For this review, take the finished solid that the model builds, in its own axes (mm). Face numbers are marked on the shaded views. Give positions to 0.01 mm unless a question says otherwise; leave off trailing zeros. Order: outer loops, then holes, each group sorted by start corner. A loop starts at its lowest first (then second) coordinate and runs counter-clockwise, first axis right, second up.
Item 1: Consider section A-A (z = 80.5). Give the boundary of the cut face in (x, y), plus the area to 3 significant figures.
Item 2: Consider section D-D (y = -23). Give the boundary of the cut face in (x, z), plus the area to 3 significant figures.
Item 3: The part is to be moulded in two halves that separate along X. For the marked faces 1, 2 and 3, say which applies: released by +X, released by -X, zero draft, split by the parting line, or undercut.
Item 4: For probe 1 along Y at (x, z) = (-0.25, 115); probe 2 along Z at (x, y) = (-0.75, -17); probe 3 along Z at (x, y) = (-11.25, -7), list the stretches that pass through material, from the lowest coordinate up.
Item 5: For P1, Ø6, axis at x = -1.5, z = 27, coming from the -Y side; P2, Ø5, axis at y = -2, z = 47.5, coming from the +X side; P3, Ø9.5, axis at x = 0, y = 0, coming from the -Z side; P4, Ø8, axis at x = 0.5, y = -3.5, coming from the +Z side, all flat-tipped, find the tip position at first contact; note any pin that passes through.
Item 6: Consider section B-B (x = 0). Give the boundary of the cut face in (y, z).
Item 7: Consider section C-C (y = 0). Give the boundary of the cut face in (x, z).
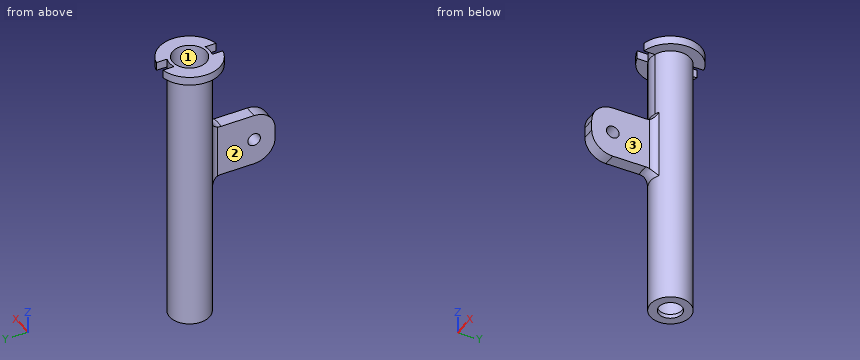
Autodesk Inventor part; units mm, degrees
ref_plane "YZ Plane" through (0, 0, 0) normal (1, 0, 0) x (0, 1, 0)
ref_plane "XZ Plane" through (0, 0, 0) normal (0, 1, 0) x (-1, 0, 0)
ref_plane "XY Plane" through (0, 0, 0) normal (0, 0, 1) x (1, 0, 0)
sketch "Boceto2" plane through (0, 0, 0) normal (0, 0, 1) x (1, 0, 0)
  circle A0 centre (0, 0) radius 9.5
  circle A1 centre (0, 0) radius 5.5
extrude "Extrusión1" add sketch "Boceto2" along normal blind 2
sketch "Boceto3" plane through (0, 0, 2) normal (0, 0, 1) x (1, 0, 0)
  circle A0 centre (0, 0) radius 9.5
  circle A1 centre (0, 0) radius 8
  dimension "d5" = 16
extrude "Extrusión2" add sketch "Boceto3" along normal blind 130
sketch "Boceto4" plane through (0, 0, 132) normal (0, 0, 1) x (1, 0, 0)
  circle A0 centre (0, 0) radius 9.5
  circle A1 centre (0, 0) radius 8
  circle A2 centre (0, 0) radius 14.5
  line L0 (3, 14.186261) -> (3, -14.186261)
  line L1 (-3, 14.186261) -> (-3, -14.186261)
  point P0 (3, 0)
  point P1 (-3, 0)
  point P2 (-3, 9.013878)
  point P3 (-3, -9.013878)
  point P4 (3, -9.013878)
  point P5 (3, 9.013878)
  dimension "d36" = 19
  dimension "d37" = 5
  dimension "d38" = 3
  dimension "d39" = 3
extrude "Extrusión3" add sketch "Boceto4" against normal blind 4 contours A0 L0 A2 | A0 L1 A2
sketch "Boceto5" plane through (0, 0, 128) normal (0, 0, -1) x (-1, 0, 0)
  line L0 (9.380832, 1.5) -> (10.897247, 1.5)
  line L1 (-9.380832, 1.5) -> (-10.897247, 1.5)
  line L2 (-9.380832, -1.5) -> (-10.897247, -1.5)
  line L3 (9.380832, -1.5) -> (10.897247, -1.5)
  arc A0 (-9.380832, 1.5) -> (-9.380832, -1.5) centre (0, 0) ccw
  arc A1 (9.380832, -1.5) -> (9.380832, 1.5) centre (0, 0) ccw
  line L4 (-10.897247, 1.5) -> (-12.409674, 1.5)
  line L5 (-10.897247, -1.5) -> (-12.409674, -1.5)
  line L6 (10.897247, 1.5) -> (12.409674, 1.5)
  line L7 (10.897247, -1.5) -> (12.409674, -1.5)
  arc A2 (-12.409674, 1.5) -> (-12.409674, -1.5) centre (0, 0) ccw
  arc A3 (12.409674, -1.5) -> (12.409674, 1.5) centre (0, 0) ccw
extrude "Extrusión4" [suppressed]
sketch "Boceto6" plane through (0, 0, 128) normal (0, 0, -1) x (-1, 0, 0)
  arc A0 (-3, -9.013878) -> (3, -9.013878) centre (0, 0) ccw
  line L0 (-2.5, -20.682789) -> (-2.5, -15.634719)
  line L1 (-3, -9.013878) -> (-3, -39.013878)
  line L2 (3, -9.013878) -> (3, -39.013878)
  line L3 (-3, -39.013878) -> (3, -39.013878)
  point P0 (-1.5, -10.897247)
  point P1 (-1.5, -9.380832)
extrude "Extrusión5" add sketch "Boceto6" along normal blind 60
sketch "Boceto7" plane through (0, 0, 128) normal (0, 0, 1) x (1, 0, 0)
  line L0 (-3, -39.013878) -> (-3, -9.013878)
  line L1 (-3, -9.013878) -> (-3, -39.013878)
  line L2 (3, -39.013878) -> (-3, -39.013878)
  line L3 (-3, -39.013878) -> (3, -39.013878)
  arc A0 (-3, -9.013878) -> (3, -9.013878) centre (0, 0) ccw
  line L4 (3, -39.013878) -> (3, -9.013878)
  circle A1 centre (0, 0) radius 9.5
extrude "Extrusión6" cut sketch "Boceto7" against normal blind 35 contours L0 A0 L4 L2
fillet "Empalme1" radius 10 2 edges at (0, -39.0139, 93) (0, -39.0139, 68)
fillet "Empalme2" radius 4 4 edges at (0, -9.5, 93) (3, -9.0139, 80.5) (-3, -9.0139, 80.5) (0, -9.5, 68)
sketch "Boceto8" plane through (3, -39.013878, 83) normal (1, 0, 0) x (0, 0, -1)
  arc A0 (-10, 10) -> (0, 0) centre (0, 10) ccw
  circle A1 centre (2.5, 10) radius 3
  point P0 (83, 39.013878)
  point P1 (15, 10)
extrude "Extrusión7" cut sketch "Boceto8" against normal blind 6
properties part number "Tubo"
Resolved:
1. outline: (-4.93, -8.12) arc R4 cw to (-3, -11.54) - (-3, -26.01) - (3, -26.01) - (3, -11.54) arc R4 cw to (4.93, -8.12) arc R9.5 ccw (long way) to start; (-3, -39.01) - (3, -39.01) - (3, -32.01) - (-3, -32.01) - close; hole circle Ø16 at (0, 0)
1. area: 226 mm2
2. outline: (-3, 68) - (3, 68) - (3, 93) - (-3, 93) - close
2. area: 150 mm2
3. face 1: undercut
3. face 2: released by -X
3. face 3: released by +X
4. probe 1: y = -9.5 to -8, 8 to 9.5
4. probe 2: z = 68 to 93
4. probe 3: z = 128 to 132
5. P1: stops at y = -9.5
5. P2: stops at x = 9.5
5. P3: passes through
5. P4: stops at z = 2
6. outline: (-39.01, 78) arc R10 ccw to (-29.01, 68) - (-13.5, 68) arc R4 cw to (-9.5, 64) - (-9.5, 0) - (-5.5, 0) - (-5.5, 2) - (-8, 2) - (-8, 132) - (-9.5, 132) - (-9.5, 97) arc R4 cw to (-13.5, 93) - (-29.01, 93) arc R10 ccw to (-39.01, 83) - close; (5.5, 0) - (9.5, 0) - (9.5, 132) - (8, 132) - (8, 2) - (5.5, 2) - close; hole circle Ø6 at (-29.01, 80.5)
7. outline: (-14.5, 128) - (-9.5, 128) - (-9.5, 0) - (-5.5, 0) - (-5.5, 2) - (-8, 2) - (-8, 132) - (-14.5, 132) - close; (5.5, 0) - (9.5, 0) - (9.5, 128) - (14.5, 128) - (14.5, 132) - (8, 132) - (8, 2) - (5.5, 2) - close
